```python
from build123d import *

# Parameters (mm, degrees)
CYLINDER004_R     = 1.7
CYLINDER004_DEPTH = 10
CYLINDER003_R     = 1.7
CYLINDER003_DEPTH = 10
BOX008_W          = 30
BOX008_H          = 5
BOX008_DEPTH      = 3


with BuildPart() as cylinder004:
    # Cylinder004 → Cylinder004 (new body)
    with BuildSketch(Plane(origin=(27, 2.5, 0), x_dir=(1, 0, 0), z_dir=(0, 0, 1))):
        Circle(CYLINDER004_R)
    extrude(amount=CYLINDER004_DEPTH)


with BuildPart() as cylinder003:
    # Cylinder003 → Cylinder003 (new body)
    with BuildSketch(Plane(origin=(3, 2.5, 0), x_dir=(1, 0, 0), z_dir=(0, 0, 1))):
        Circle(CYLINDER003_R)
    extrude(amount=CYLINDER003_DEPTH)


with BuildPart() as obj1:
    # Box008 → Box008 (new body)
    with BuildSketch(Plane.XY):
        with Locations((15, 2.5)):
            Rectangle(BOX008_W, BOX008_H)
    extrude(amount=BOX008_DEPTH)

    # Cut006: cut Cylinder003
    add(cylinder003.part, mode=Mode.SUBTRACT)

    # Cut007: cut Cylinder004
    add(cylinder004.part, mode=Mode.SUBTRACT)


solid = obj1.part
```
Read the model definition and answer for the solid it produces. Units are mm, in the model's axes. Coordinates: 2 decimals unless noted, no trailing zeros. Loops run counter-clockwise (first coordinate to the right, second up) from the corner with the lowest first, then second, coordinate; pieces in that order, holes last. Notation, with made-up numbers: (61.25, 19.25) - (108.25, 19.25) arc R20 ccw to (108.25, 57.25) - close; hole circle Ø2 at (-6, 82). An arc over 180 degrees is marked (long way). Answer in a Markdown table with one row per item.
1. Find section B-B, the plane y = 2.5. Write down the section's boundary in (x, z).
Conclusion:
| item | result |
|---|---|
| outline | (0, 0) - (1.3, 0) - (1.3, 3) - (0, 3) - close; (4.7, 0) - (25.3, 0) - (25.3, 3) - (4.7, 3) - close; (28.7, 0) - (30, 0) - (30, 3) - (28.7, 3) - close |
2. Find section C-C, the plane z = 1.95. Write down the section's boundary in (x, y), then the cut area to 3 significant figures.
Conclusion:
| item | result |
|---|---|
| outline | (0, 0) - (30, 0) - (30, 5) - (0, 5) - close; hole circle Ø3.4 at (3, 2.5); hole circle Ø3.4 at (27, 2.5) |
| area | 132 mm² |
3. Find section D-D, the plane y = 1.05. Write down the section's boundary in (x, z), then the cut area to 3 significant figures.
Conclusion:
| item | result |
|---|---|
| outline | (0, 0) - (2.11, 0) - (2.11, 3) - (0, 3) - close; (3.89, 0) - (26.11, 0) - (26.11, 3) - (3.89, 3) - close; (27.89, 0) - (30, 0) - (30, 3) - (27.89, 3) - close |
| area | 79.4 mm² |
4. Determine the mould class of faces 1 (the face through (4.62, 3.01, 1.48)), 2 (the face through (30, 2, 1)), 3 (the face through (15, 3, 3)) for opening direction X: +X half, -X half, draft (parallel to the pull), parting line (faces both ways), or undercut.
Conclusion:
| item | result |
|---|---|
| face 1 | undercut |
| face 2 | +X half |
| face 3 | draft |
5. Find section A-A, the plane x = 3. Write down the section's boundary in (y, z).
Conclusion:
| item | result |
|---|---|
| outline | (0, 0) - (0.8, 0) - (0.8, 3) - (0, 3) - close; (4.2, 0) - (5, 0) - (5, 3) - (4.2, 3) - close |
6. Straight lines are drawn through the part: line 1 (X direction, y = 2.5, z = 0.6); line 2 (Y direction, x = 3, z = 1.25); line 3 (X direction, y = 3.05, z = 0.15). For each, find the intervals that lie inside material, in ascending order.
Conclusion:
| item | result |
|---|---|
| line 1 | x = 0 to 1.3, 4.7 to 25.3, 28.7 to 30 |
| line 2 | y = 0 to 0.8, 4.2 to 5 |
| line 3 | x = 0 to 1.39, 4.61 to 25.39, 28.61 to 30 |
